CAD build for the part. Positions are in the model's coordinates, mm. A direction names the side the tool comes from. Round coordinates to 2 decimals unless told otherwise and drop trailing zeros. Loops run counter-clockwise (first coordinate to the right, second up) from the corner with the lowest first, then second, coordinate; pieces in that order, holes last. Notation, with made-up numbers: M 61,16 L 112,16 A24 ccw 112,46 Z; hole C -34.75,37 d11. An arc over 180 degrees is marked long. Use a Markdown table: item, result. Add a question column.
(1) Flat gauge pins, fed straight in: P1, Ø5, axis at y = 21.22, z = 4.76, coming from the -X side; P2, Ø4, axis at y = 52.2, z = 4.76, coming from the +X side; P3, Ø1.5, axis at x = 1.5, z = 4.5, coming from the -Y side. Where does each tip first touch, or does it go through?
(2) Wall check: L1, parallel to X at y = -20.5, z = 8; L2, parallel to Y at x = 0, z = 8.5; L3, parallel to Z at x = -1.9, y = 21.5 (3 decimals). Give the ranges that are in metal, low to high.
(3) Two-plate mould, pull along Y, no slides. Class faces 1 (the face through (-2.32, 15.06, 4.7)), 2 (the face through (-0.885, -25, 5)), 3 (the face through (2.02, 12.32, 4.7)): released by +Y, released by -Y, zero draft, split by the parting line, or undercut.
(4) Band-saw the part on A-A, the plane y = 8. Write the cut outline in (x, z) (3 decimals), and give its area (3 significant figures).
(5) Which spindle directions (+Z, -Z, +X, -X, +Y, -Y) get a long thin tool onto all of the face, cutting with end or side? Do faces 4 (the face through (-0.885, 36, 5)), 5 (the face through (1, 6, 0)), 6 (the face through (0.581, 9.4, 3.6)). Say none if no direction does.
(6) Band-saw the part on B-B, the plane y = 37.5. Write the cut outline in (x, z) (3 decimals).
from build123d import *

# Parameters (mm, degrees)
F1_DEPTH = 9.525
F2_R     = 1.8288
F2_R_2   = 3.175
F3_DEPTH = 4.88442
F4_R     = 0.762


with BuildPart() as f1:
    # F0 (on Top) → F1 (new body)
    with BuildSketch(Plane.XY):
        with BuildLine():
            ThreePointArc((0.581024, 1.402716), (0.430021, 0.643572), (0, 0))
            Line((0, 0), (-1.512274, -1.512274))
            ThreePointArc((-1.512274, -1.512274), (-2.312851, -2.710422), (-2.593976, -4.123733))
            Line((-2.593976, -4.123733), (-2.593976, -44.634784))
            Line((-2.593976, -44.634784), (-0.884556, -44.634784))
            Line((-0.884556, -44.634784), (-0.884556, -4.123733))
            ThreePointArc((-0.884556, -4.123733), (-0.733553, -3.364588), (-0.303532, -2.721017))
            Line((-0.303532, -2.721017), (1.208743, -1.208742))
            ThreePointArc((1.208743, -1.208742), (2.009319, -0.010595), (2.290444, 1.402716))
            Line((2.290444, 1.402716), (2.290444, 10.927716))
            ThreePointArc((2.290444, 10.927716), (2.009319, 12.341027), (1.208743, 13.539175))
            Line((1.208743, 13.539175), (-0.303532, 15.051449))
            ThreePointArc((-0.303532, 15.051449), (-0.733553, 15.695021), (-0.884556, 16.454165))
            Line((-0.884556, 16.454165), (-0.884556, 56.965216))
            Line((-0.884556, 56.965216), (-2.593976, 56.965216))
            Line((-2.593976, 56.965216), (-2.593976, 16.454165))
            ThreePointArc((-2.593976, 16.454165), (-2.312851, 15.040854), (-1.512274, 13.842707))
            Line((-1.512274, 13.842707), (0, 12.330432))
            ThreePointArc((0, 12.330432), (0.430021, 11.686861), (0.581024, 10.927716))
            Line((0.581024, 10.927716), (0.581024, 1.402716))
        make_face()
    extrude(amount=F1_DEPTH)

    # F2 (on face) → F3 (cut, through all)
    with BuildSketch(Plane(origin=(-2.593976, 0, 0), x_dir=(0, -1, 0), z_dir=(-1, 0, 0))):
        with Locations((-52.202716, 4.7625)):
            Circle(F2_R)
        with Locations((-21.216665, 4.7625)):
            Circle(F2_R)
        with Locations((8.886233, 4.7625)):
            Circle(F2_R)
        with Locations((39.872284, 4.7625)):
            Circle(F2_R)
        with Locations((-6.165216, 4.7625)):
            Circle(F2_R_2)
    extrude(amount=-F3_DEPTH, mode=Mode.SUBTRACT)

    # F4
    f4_edges = [f1.edges().sort_by_distance(p)[0] for p in [
        (-1.739266, 56.965216, 9.525),
        (-1.739266, 56.965216, 0),
        (-1.739266, -44.634784, 9.525),
        (-1.739266, -44.634784, 0),
    ]]
    fillet(f4_edges, radius=F4_R)


solid = f1.part
Return value:
| question | item | result |
|---|---|---|
| 1 | P1 | x = -2.59 |
| 1 | P2 | x = -0.88 |
| 1 | P3 | y = -1.67 |
| 2 | L1 | -2.59 to -0.88 |
| 2 | L2 | -2.42 to 0, 12.33 to 14.75 |
| 2 | L3 | 0 to 2.956, 6.569 to 9.525 |
| 3 | face 1 | undercut |
| 3 | face 2 | zero draft |
| 3 | face 3 | released by +Y |
| 4 | outline | M 0.581,0 L 2.29,0 L 2.29,2.171 L 0.581,2.171 Z; M 0.581,7.354 L 2.29,7.354 L 2.29,9.525 L 0.581,9.525 Z |
| 4 | area | 7.42 mm^2 |
| 5 | face 4 | +Z, -Z, +X, +Y |
| 5 | face 5 | -Z, +X, -X, +Y, -Y |
| 5 | face 6 | +Z, -Z, -X |
| 6 | outline | M -2.594,0 L -0.885,0 L -0.885,9.525 L -2.594,9.525 Z |
